Read the model definition and answer for the solid it produces. Units are mm, in the model's axes. Face numbers are marked on the shaded views. Coordinates: 2 decimals unless noted, no trailing zeros. Order: outer loops, then holes, each group sorted by start corner. A loop starts at its lowest first (then second) coordinate and runs counter-clockwise, first axis right, second up.
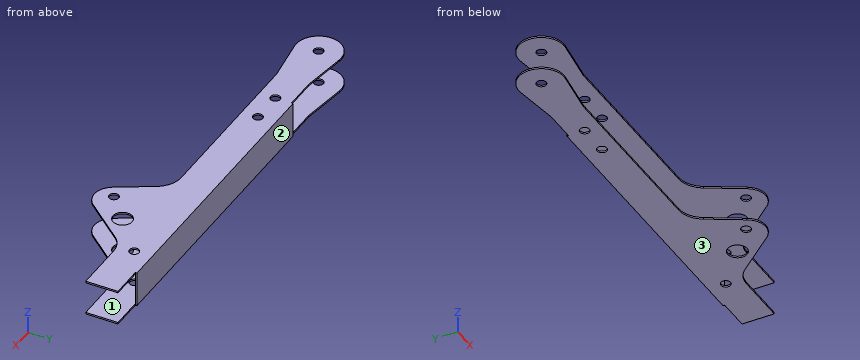
```python
from build123d import *

# Parameters (mm, degrees)
SKETCH_1_R      = 1.5
SKETCH_1_R_2    = 3
EXTRUDE_1_DEPTH = 0.5
SKETCH_3_R      = 3
SKETCH_3_R_2    = 1.5
EXTRUDE_2_DEPTH = 0.5
SKETCH_4_W      = 90
SKETCH_4_H      = 11
EXTRUDE_3_DEPTH = 0.5
FILLET_1_R      = 8
FILLET_2_R      = 6


with BuildPart() as part:
    # Sketch 1 → Extrude 1 (new body)
    with BuildSketch(Plane.XY):
        with BuildLine():
            Line((-28.937588447, 12.863865809), (81.062411553, 12.863865809))
            Line((81.062411553, 12.863865809), (81.062411553, 2.863865809))
            Line((81.062411553, 2.863865809), (61.338833841, 2.863865809))
            Line((61.338833841, 2.863865809), (43.106996214, -18.863992184))
            Line((43.106996214, -18.863992184), (30.562411553, 2.863865809))
            Line((30.562411553, 2.863865809), (-28.937588447, 2.863865809))
            Line((-28.937588447, 2.863865809), (-42.98243101, 0.92933812))
            ThreePointArc((-42.98243101, 0.92933812), (-50.937588447, 7.863865809), (-42.98243101, 14.798393498))
            Line((-42.98243101, 14.798393498), (-28.937588447, 12.863865809))
        make_face()
        with Locations((-43.937588447, 7.863865809)):
            Circle(SKETCH_1_R, mode=Mode.SUBTRACT)
        with Locations((42.562411553, -9.136134191)):
            Circle(SKETCH_1_R, mode=Mode.SUBTRACT)
        with Locations((50.562411553, -2.136134191)):
            Circle(SKETCH_1_R_2, mode=Mode.SUBTRACT)
        with Locations((-18.937588447, 7.863865809)):
            Circle(SKETCH_1_R, mode=Mode.SUBTRACT)
        with Locations((-8.937588447, 7.863865809)):
            Circle(SKETCH_1_R, mode=Mode.SUBTRACT)
        with Locations((62.409410938, 7.863865809)):
            Circle(SKETCH_1_R, mode=Mode.SUBTRACT)
    extrude(amount=EXTRUDE_1_DEPTH)



with BuildPart() as body_2:
    # Sketch 3 → Extrude 2 (new body)
    with BuildSketch(Plane.XY.offset(-10)):
        with BuildLine():
            Line((43.106996214, -18.863992184), (61.338833841, 2.863865809))
            Line((61.338833841, 2.863865809), (81.062411553, 2.863865809))
            Line((81.062411553, 2.863865809), (81.062411553, 12.863865809))
            Line((81.062411553, 12.863865809), (-28.937588447, 12.863865809))
            Line((-28.937588447, 12.863865809), (-42.98243101, 14.798393498))
            ThreePointArc((-42.98243101, 14.798393498), (-50.937588447, 7.863865809), (-42.98243101, 0.92933812))
            Line((-42.98243101, 0.92933812), (-28.937588447, 2.863865809))
            Line((-28.937588447, 2.863865809), (30.562411553, 2.863865809))
            Line((30.562411553, 2.863865809), (43.106996214, -18.863992184))
        make_face()
        with Locations((50.562411553, -2.136134191)):
            Circle(SKETCH_3_R, mode=Mode.SUBTRACT)
        with Locations((42.562411553, -9.136134191)):
            Circle(SKETCH_3_R_2, mode=Mode.SUBTRACT)
        with Locations((-43.937588447, 7.863865809)):
            Circle(SKETCH_3_R_2, mode=Mode.SUBTRACT)
        with Locations((62.409410938, 7.863865809)):
            Circle(SKETCH_3_R_2, mode=Mode.SUBTRACT)
        with Locations((-8.937588447, 7.863865809)):
            Circle(SKETCH_3_R_2, mode=Mode.SUBTRACT)
        with Locations((-18.937588447, 7.863865809)):
            Circle(SKETCH_3_R_2, mode=Mode.SUBTRACT)
    extrude(amount=-EXTRUDE_2_DEPTH)


with BuildPart() as part_1:
    add(part.part)

    add(body_2.part)  # Extrude 3 merges body 2
    # Sketch 4 → Extrude 3 (add)
    with BuildSketch(Plane(origin=(0, 12.863865809, 0), x_dir=(1, 0, 0), z_dir=(0, 1, 0))):
        with Locations((26.062411553, 5)):
            Rectangle(SKETCH_4_W, SKETCH_4_H)
    extrude(amount=EXTRUDE_3_DEPTH)

    # Fillet 1
    fillet_1_edges = [part_1.edges().sort_by_distance(p)[0] for p in [
        (61.338833841, 2.863865809, 0.25),
        (30.562411553, 2.863865809, 0.25),
        (30.562411553, 2.863865809, -10.25),
        (61.338833841, 2.863865809, -10.25),
    ]]
    fillet(fillet_1_edges, radius=FILLET_1_R)

    # Fillet 2
    fillet_2_edges = [part_1.edges().sort_by_distance(p)[0] for p in [
        (43.106996214, -18.863992184, 0.25),
        (43.106996214, -18.863992184, -10.25),
    ]]
    fillet(fillet_2_edges, radius=FILLET_2_R)


solid = part_1.part
```
1) A cutting plane is placed at D-D, the plane x = 56. Determine the outline of the cut face in (y, z), and give its area (3 significant figures).
A:
outline: (-3.5, -10.5) - (13.36, -10.5) - (13.36, 0.5) - (-3.5, 0.5) - (-3.5, 0) - (12.86, 0) - (12.86, -10) - (-3.5, -10) - close
area: 21.9 mm2
2) Flat-ended cylindrical pins translate along their axes: pin 1 Ø0.6 at (x, z) = (-26, -10.5) entering from +Y; pin 2 Ø6 at (y, z) = (-10.5, -8) entering from -X. Find the tip coordinate at first contact, or state that the pin passes through.
A:
pin 1: stops at y = 12.86
pin 2: stops at x = 36.99
3) A cutting plane is placed at C-C, the plane z = -5.25. Determine the outline of the cut face in (x, y).
A:
outline: (-18.94, 12.86) - (71.06, 12.86) - (71.06, 13.36) - (-18.94, 13.36) - close
4) Straight lines are drawn through the part: line 1 (Z direction, x = 53.5, y = -3.5); line 2 (Y direction, x = 22.5, z = -5); line 3 (X direction, y = 13, z = -3.5). For each, find the intervals that lie inside material, in ascending order.
A:
line 1: z = -10.5 to -10, 0 to 0.5
line 2: y = 12.86 to 13.36
line 3: x = -18.94 to 71.06
5) Determine the mould class of the marked faces 1, 2 and 3 for opening direction Z: pulls with the +Z half, pulls with the -Z half, needs draft (parallel to the pull), parting line crosses it, or undercut.
A:
face 1: undercut
face 2: needs draft
face 3: pulls with the -Z half
6) A cutting plane is placed at A-A, the plane y = 5. Determine the outline of the cut face in (x, z), and give its area (3 significant figures).
A:
outline: (-50.32, -10.5) - (81.06, -10.5) - (81.06, -10) - (-50.32, -10) - close; (-50.32, 0) - (81.06, 0) - (81.06, 0.5) - (-50.32, 0.5) - close
area: 131 mm2
7) A cutting plane is placed at B-B, the plane x = 8. Determine the outline of the cut face in (y, z).
A:
outline: (2.86, -10.5) - (13.36, -10.5) - (13.36, 0.5) - (2.86, 0.5) - (2.86, 0) - (12.86, 0) - (12.86, -10) - (2.86, -10) - close
